Source: CAD feature listing. Evaluate the final solid. Frame: model axes, mm. A direction names the side the tool comes from. Coordinates: 2 decimals unless noted, no trailing zeros. Order: outer loops, then holes, each group sorted by start corner. A loop starts at its lowest first (then second) coordinate and runs counter-clockwise, first axis right, second up. Notation, with made-up numbers: (24, 68.25) -> (51, 68.25) arc R7 cw to (51, 81.25) -> close; hole circle Ø11 at (18, 8). An arc over 180 degrees is marked (long way). Write item = value, one per line. Start each with the question number.
Item 1: Section query C-C (y = -1.3). Output: boundary loops of the cut face in (x, z) (3 decimals), then the cut area to 3 significant figures.
Item 2: Mould query, pull axis Z, two halves, no side actions, for faces 6 (the flat face through (127.405, -1.002, 37.445)), 7 (the flat face through (4.91, -1, -34.96)), 8 (the flat face through (132.945, -1.002, -22.223)). Classes: released by +Z, released by -Z, zero draft, split by the parting line, or undercut.
Item 3: Contact query for a flat-ended pin moving along its axis: pin 1 (1 mm diameter, centred on x = -4.5, y = -1, fed in from +Z). Output: stop coordinate, or through.
Item 4: Section query A-A (x = 98). Output: boundary loops of the cut face in (y, z).
Item 5: Set-up query: faces 1 (the flat face through (105.38, -1.002, 5.267)), 2 (the flat face through (80.148, -1.002, -32.393)), 3 (the flat face through (-13.94, -1, 8.05)), 4 (the flat face through (127.04, -1, -37.56)), 5 (the flat face through (5.291, -1.002, 34.742)). Return all of +Z, -Z, +X, -X, +Y, -Y with unobstructed straight access to the full face (end or side cutting, diameter ignored); none if empty.
Item 6: Ray query, line 1 along Z through (x, y) = (98.5, -0.55); line 2 along Z through (x, y) = (113, -1.6); line 3 along Z through (x, y) = (36.5, -0.15). Return the intervals inside material, ascending. Write a range as [from, to].
Item 7: Section query B-B (z = -29). Output: boundary loops of the cut face in (x, y).
Item 8: Section query D-D (z = 4). Output: boundary loops of the cut face in (x, y).
```python
from build123d import *

# Parameters (mm, degrees)
F1_DEPTH = 2.032


with BuildPart() as f1:
    # F0 (on Front) → F1 (new body)
    with BuildSketch(Plane.XZ):
        with BuildLine():
            Line((-27.496307, 15.875), (0, 0))
            Line((0, 0), (-27.496307, -15.875))
            Line((-27.496307, -15.875), (-35.611604, -41.613436))
            Line((-35.611604, -41.613436), (-8.64979, -42.790614))
            Line((-8.64979, -42.790614), (18.846516, -26.915614))
            ThreePointArc((18.846516, -26.915614), (32.532451, -22.474943), (46.885606, -23.48057))
            Line((46.885606, -23.48057), (114.355525, -41.55908))
            Line((114.355525, -41.55908), (140.093962, -33.443783))
            Line((140.093962, -33.443783), (125.593588, -10.682756))
            Line((125.593588, -10.682756), (85.725, 0))
            Line((85.725, 0), (125.593588, 10.682756))
            Line((125.593588, 10.682756), (140.093962, 33.443783))
            Line((140.093962, 33.443783), (114.355525, 41.55908))
            Line((114.355525, 41.55908), (46.885606, 23.48057))
            ThreePointArc((46.885606, 23.48057), (32.532451, 22.474943), (18.846516, 26.915614))
            Line((18.846516, 26.915614), (-8.64979, 42.790614))
            Line((-8.64979, 42.790614), (-35.611604, 41.613436))
            Line((-35.611604, 41.613436), (-27.496307, 15.875))
        make_face()
    extrude(amount=F1_DEPTH)


solid = f1.part
```
Computed:
q1.outline = (-35.612, -41.613) -> (-8.65, -42.791) -> (18.847, -26.916) arc R37.73 cw to (46.886, -23.481) -> (114.356, -41.559) -> (140.094, -33.444) -> (125.594, -10.683) -> (85.725, 0) -> (125.594, 10.683) -> (140.094, 33.444) -> (114.356, 41.559) -> (46.886, 23.481) arc R37.73 cw to (18.847, 26.916) -> (-8.65, 42.791) -> (-35.612, 41.613) -> (-27.496, 15.875) -> (0, 0) -> (-27.496, -15.875) -> close
q1.area = 9,850 mm^2
q2.face_6 = released by +Z
q2.face_7 = released by -Z
q2.face_8 = undercut
q3.pin_1 = 40.68
q4.outline = (-2.03, -37.18) -> (0, -37.18) -> (0, -3.29) -> (-2.03, -3.29) -> close; (-2.03, 3.29) -> (0, 3.29) -> (0, 37.18) -> (-2.03, 37.18) -> close
q5.face_1 = +X, +Y, -Y
q5.face_2 = -Z, +Y, -Y
q5.face_3 = -X, +Y, -Y
q5.face_4 = -Z, +X, +Y, -Y
q5.face_5 = +Z, +Y, -Y
q6.line_1 = [-37.31, -3.42], [3.42, 37.31]
q6.line_2 = [-41.2, -7.31], [7.31, 41.2]
q6.line_3 = [-22.2, 22.2]
q7.outline = (-31.63, -2.03) -> (15.24, -2.03) -> (15.24, 0) -> (-31.63, 0) -> close; (67.48, -2.03) -> (137.26, -2.03) -> (137.26, 0) -> (67.48, 0) -> close
q8.outline = (-6.93, -2.03) -> (100.65, -2.03) -> (100.65, 0) -> (-6.93, 0) -> close
